```python
from build123d import *

# Parameters (mm, degrees)
SKETCH_R           = 98.425
PAD_DEPTH          = 0.6
PAD001_DEPTH       = 5
POLARPATTERN_COUNT = 4
SKETCH002_R        = 28
POCKET_DEPTH       = 5.601
SKETCH003_W        = 15
SKETCH003_H        = 24
POCKET001_DEPTH    = 5.601


with BuildPart() as part:
    # Sketch → Pad (new body)
    with BuildSketch(Plane.XY):
        Circle(SKETCH_R)
    extrude(amount=-PAD_DEPTH)

    # Sketch001 → Pad001 (new body)
    with BuildSketch(Plane.XY):
        with BuildLine():
            ThreePointArc((3.175, -21.997045), (15.715448, -15.715448), (21.997045, -3.175))
            Line((21.997045, -3.175), (98.373777, -3.175))
            ThreePointArc((3.175, -98.373777), (69.596985, -69.596985), (98.373777, -3.175))
            Line((3.175, -21.997045), (3.175, -98.373777))
        make_face()
    pad001 = extrude(amount=PAD001_DEPTH)

    # PolarPattern: Pad001 ×4 about axis
    polarpattern_axis = Axis((0, 0, 0), (0, 0, 1))
    for i in range(1, POLARPATTERN_COUNT):
        add(pad001.rotate(polarpattern_axis, i * 360 / POLARPATTERN_COUNT))

    # Sketch002 → Pocket (cut, through all)
    with BuildSketch(Plane.XY.offset(5)):
        Circle(SKETCH002_R)
    extrude(amount=-POCKET_DEPTH, mode=Mode.SUBTRACT)

    # Sketch003 → Pocket001 (cut, through all)
    with BuildSketch(Plane(origin=(0, 0, -0.6), x_dir=(1, 0, 0), z_dir=(0, 0, -1))):
        with Locations((97.5, 0)):
            Rectangle(SKETCH003_W, SKETCH003_H)
    extrude(amount=-POCKET001_DEPTH, mode=Mode.SUBTRACT)


solid = part.part
```
Read the model definition and answer for the solid it produces. Units are mm, in the model's axes. A direction names the side the tool comes from. Give positions to 0.01 mm unless a question says otherwise; leave off trailing zeros. Order: outer loops, then holes, each group sorted by start corner. A loop starts at its lowest first (then second) coordinate and runs counter-clockwise, first axis right, second up. Notation, with made-up numbers: (66.5, 71.25) -> (114.5, 71.25) arc R15 ccw to (114.5, 76.25) -> close; hole circle Ø11 at (50, 76). An arc over 180 degrees is marked (long way). One line per item, written item: value. Start each with the question number.
(1) The part is cut by section D-D (y = -23). Determine the outline of the cut face in (x, z).
(2) The part is cut by section A-A (x = 0). Determine the outline of the cut face in (y, z) (3 decimals).
(3) Straight lines are drawn through the part: L1, parallel to X at y = 3.5, z = 2.5; L2, parallel to Y at x = 60, z = 0.1 (3 decimals); L3, parallel to Y at x = -16, z = -0.3. For each, find the intervals that lie inside material, in ascending order.
(4) The part is cut by section C-C (y = 0). Determine the outline of the cut face in (x, z) (3 decimals).
(5) A tool of negligible diameter and unlimited length cuts with its end or side. For faces 5 (the flat face through (94, -12, 2)), 6 (the flat face through (0, 64, 0)), 7 (the flat face through (58, -3.175, 2)), from which of +Z, -Z, +X, -X, +Y, -Y can it reach the whole face along a straight path? Write none if from no direction.
(6) For a pull along X with two mould halves and no side action, classify faces 1 (the flat face through (-3.175, 63, 2)), 2 (the cylindrical face through (25.865, -10.724, 2.239)), 3 (the flat face through (90, 0.2, -0.3)), 4 (the flat face through (39, 51, 5)) as released by +X, released by -X, zero draft, split by the parting line, or undercut.
(7) Flat-ended cylindrical pins translate along their axes: P1, Ø1.9, axis at x = 47, y = -1, coming from the +Z side; P2, Ø1, axis at x = 71.5, z = 1, coming from the +Y side; P3, Ø3, axis at x = -6.5, z = 0.5, coming from the -Y side. Find the tip coordinate at first contact, or state that the pin passes through.
(8) The part is cut by section B-B (z = 3.7). Determine the outline of the cut face in (x, y) (3 decimals), and give its area (3 significant figures).
Taken from the geometry:
1. outline: (-95.7, -0.6) -> (-15.97, -0.6) -> (-15.97, 5) -> (-95.7, 5) -> close; (15.97, -0.6) -> (95.7, -0.6) -> (95.7, 5) -> (15.97, 5) -> close
2. outline: (-98.425, -0.6) -> (-28, -0.6) -> (-28, 0) -> (-98.425, 0) -> close; (28, -0.6) -> (98.425, -0.6) -> (98.425, 0) -> (28, 0) -> close
3. L1: -98.36 to -27.78, 27.78 to 90
3. L2: -78.022 to -3.175, 3.175 to 78.022
3. L3: -97.12 to -22.98, 22.98 to 97.12
4. outline: (-98.425, -0.6) -> (-28, -0.6) -> (-28, 0) -> (-98.425, 0) -> close; (28, -0.6) -> (90, -0.6) -> (90, 0) -> (28, 0) -> close
5. face 5: +Z, -Z, +X
5. face 6: +Z, +Y, -Y
5. face 7: +Z, +X, -X
6. face 1: undercut
6. face 2: undercut
6. face 3: released by +X
6. face 4: zero draft
7. P1: z = 0
7. P2: y = 68.17
7. P3: y = -98.3
8. outline: (-98.374, -3.175) arc R98.425 ccw to (-3.175, -98.374) -> (-3.175, -27.819) arc R28 cw to (-27.819, -3.175) -> close; (-98.374, 3.175) -> (-27.819, 3.175) arc R28 cw to (-3.175, 27.819) -> (-3.175, 98.374) arc R98.425 ccw to start; (3.175, -98.374) arc R98.425 ccw to (97.691, -12) -> (90, -12) -> (90, -3.175) -> (27.819, -3.175) arc R28 cw to (3.175, -27.819) -> close; (3.175, 27.819) arc R28 cw to (27.819, 3.175) -> (90, 3.175) -> (90, 12) -> (97.691, 12) arc R98.425 ccw to (3.175, 98.374) -> close
8. area: 26,000 mm^2
